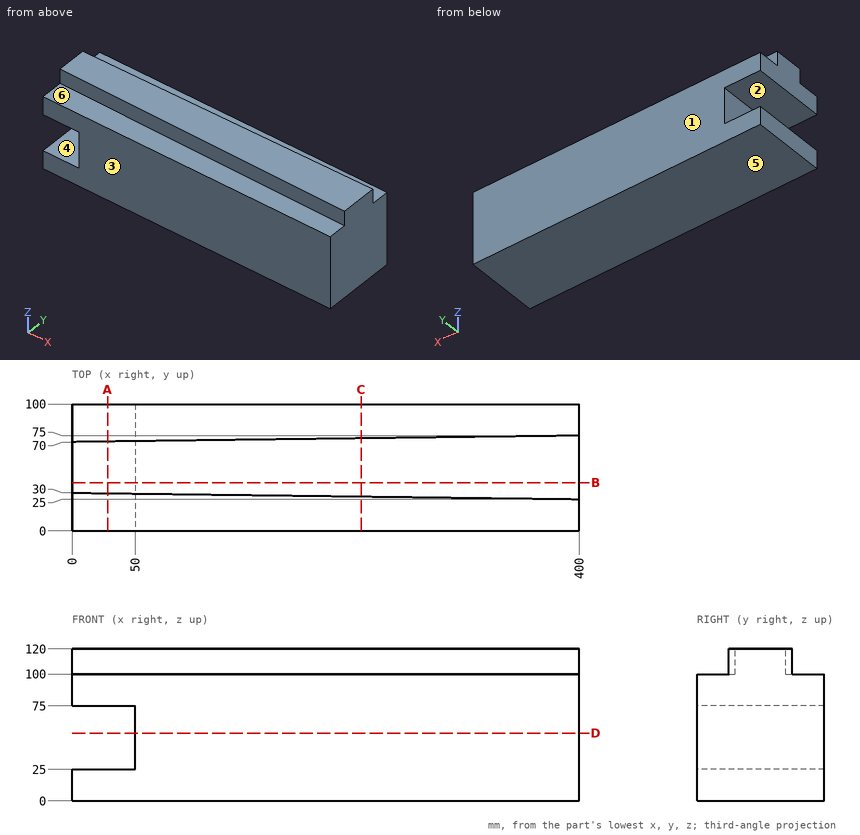
Print and shaded views of the part. All mm, measured from the part's lowest x, y and z. A direction names the side the tool comes from. Coordinates: 2 decimals unless noted, no trailing zeros. Write each loop counter-clockwise with the first axis right and the second up, starting at its lowest first coordinate (ties: lowest second). Pieces come first, ordered by that corner, then holes. Notation, with made-up numbers: M -7.75,31 L 1.25,31 A18 ccw 1.25,62 Z; hole C 81,-4 d10. An arc over 180 degrees is marked long. Return JSON: item names as keys, results as strings.
1. Saw through at C-C, the plane x = 228. Write the cut outline in (y, z), then the cut area to 3 significant figures.
Determined:
{"outline": "M 0,0 L 100,0 L 100,100 L 72.85,100 L 72.85,120 L 27.15,120 L 27.15,100 L 0,100 Z", "area": "10,900 mm²"}
2. Probe L1, parallel to Z at x = 41, y = 35; L2, parallel to X at y = 36, z = 41.5; L3, parallel to Z at x = 67, y = 22.5. List the from-to ranges inside material, lowest first.
Determined:
{"L1": "0 to 25, 75 to 120", "L2": "50 to 400", "L3": "0 to 100"}
3. 3-axis set-ups, long thin cutter, end or side, ignore diameter. For the marked faces 1 and 2: which of +Z, -Z, +X, -X, +Y, -Y reach the whole face in a straight line?
Determined:
{"face 1": "+Z, -Z, +X, -X, +Y", "face 2": "-X, +Y, -Y"}
4. Saw through at B-B, the plane y = 38. Write the cut outline in (x, z), then the cut area to 3 significant figures.
Determined:
{"outline": "M 0,0 L 400,0 L 400,120 L 0,120 L 0,75 L 50,75 L 50,25 L 0,25 Z", "area": "45,500 mm²"}
5. Flat gauge pins, fed straight in: pin 1 Ø24 at (x, y) = (101.5, 81) entering from +Z; pin 2 Ø25 at (y, z) = (66.5, 49.5) entering from -X; pin 3 Ø15 at (x, y) = (198.5, 12) entering from +Z. Where does each tip first touch, or does it go through?
Determined:
{"pin 1": "z = 120", "pin 2": "x = 50", "pin 3": "z = 100"}
6. Saw through at D-D, the plane z = 53.5. Write the cut outline in (x, y), then the cut area to 3 significant figures.
Determined:
{"outline": "M 50,0 L 400,0 L 400,100 L 50,100 Z", "area": "35,000 mm²"}
7. Saw through at A-A, the plane x = 28. Write the cut outline in (y, z).
Determined:
{"outline": "M 0,0 L 100,0 L 100,25 L 0,25 Z; M 0,75 L 100,75 L 100,100 L 70.35,100 L 70.35,120 L 29.65,120 L 29.65,100 L 0,100 Z"}
8. Pull direction Z, two halves, no side cores. Call the marked faces 3, 4, 5 and 6: pulls with the +Z half, pulls with the -Z half, needs draft (parallel to the pull), parting line crosses it, or undercut.
Determined:
{"face 3": "needs draft", "face 4": "undercut", "face 5": "pulls with the -Z half", "face 6": "pulls with the +Z half"}
